```python
from build123d import *

# Parameters (mm, degrees)
SKETCH1_R           = 6
BOSS_EXTRUDE1_DEPTH = 8
SKETCH3_R           = 7.5
BOSS_EXTRUDE2_DEPTH = 20
SKETCH4_R           = 7.5
BOSS_EXTRUDE3_DEPTH = 2.5


with BuildPart() as part:
    # Sketch1 → Boss-Extrude1 (new body)
    with BuildSketch(Plane(origin=(0, 0, 0), x_dir=(1, 0, 0), z_dir=(0, 1, 0))):
        Circle(SKETCH1_R)
    extrude(amount=BOSS_EXTRUDE1_DEPTH)

    # Sketch3 → Boss-Extrude2 (add)
    with BuildSketch(Plane.XZ):
        Circle(SKETCH3_R)
    extrude(amount=BOSS_EXTRUDE2_DEPTH)

    # Sketch4 → Boss-Extrude3 (add)
    with BuildSketch(Plane(origin=(0, 8, 0), x_dir=(1, 0, 0), z_dir=(0, 1, 0))):
        Circle(SKETCH4_R)
    extrude(amount=-BOSS_EXTRUDE3_DEPTH)


solid = part.part
```
Input: part model. Units: mm. Frame: model coordinates. A direction names the side the tool comes from. Round coordinates to 2 decimals unless told otherwise and drop trailing zeros. Loops run counter-clockwise (first coordinate to the right, second up) from the corner with the lowest first, then second, coordinate; pieces in that order, holes last.
1) Section query A-A on z = 0. Return the cut outline in (x, y).
Ans:
outline: (-7.5, -20) - (7.5, -20) - (7.5, 0) - (6, 0) - (6, 5.5) - (7.5, 5.5) - (7.5, 8) - (-7.5, 8) - (-7.5, 5.5) - (-6, 5.5) - (-6, 0) - (-7.5, 0) - close
2) Section query B-B on x = 0. Return the cut outline in (y, z), plus the area to 4 significant figures.
Ans:
outline: (-20, -7.5) - (0, -7.5) - (0, -6) - (5.5, -6) - (5.5, -7.5) - (8, -7.5) - (8, 7.5) - (5.5, 7.5) - (5.5, 6) - (0, 6) - (0, 7.5) - (-20, 7.5) - close
area: 403.5 mm2
3) Material intervals for line 1 (Z direction, x = -4.5, y = -8.75); line 2 (Y direction, x = -6.25, z = -4), sorted ascending.
Ans:
line 1: z = -6 to 6
line 2: y = -20 to 0, 5.5 to 8
4) Set-up query: faces 1 (the flat face through (0, 8, 0)), 2 (the cylindrical face through (-6, 3, 0)). Return all of +Z, -Z, +X, -X, +Y, -Y with unobstructed straight access to the full face (end or side cutting, diameter ignored); none if empty.
Ans:
face 1: +Z, -Z, +X, -X, +Y
face 2: none
5) Pin query (flat end, axial travel): pin 1 (4 mm diameter, centred on x = -2, y = 1, fed in from +Z); pin 2 (1 mm diameter, centred on y = -12.5, z = -2, fed in from +X); pin 3 (2 mm diameter, centred on x = 3.5, y = 4, fed in from -Z). Return the tip coordinate at first contact, or that it passes through.
Ans:
pin 1: stops at z = 7.5
pin 2: stops at x = 7.35
pin 3: stops at z = -5.45
6) Pull-direction query (Y, two-part tool) for faces 3 (the flat face through (2, 0, 6)), 4 (the cylindrical face through (-7.493, 6.768, -0.33)), 5 (the flat face through (0, -20, 0)); classes: released by +Y, released by -Y, zero draft, split by the parting line, or undercut.
Ans:
face 3: undercut
face 4: zero draft
face 5: released by -Y
7) Section query C-C on y = -0.75. Return the cut outline in (x, z).
Ans:
outline: circle Ø15 at (0, 0)
